Could you check a few things on this drawing? It's one solid part, dimensions in mm from its lowest x, y, z. Give positions to 0.01 mm unless a question says otherwise; leave off trailing zeros. Order: outer loops, then holes, each group sorted by start corner. A loop starts at its lowest first (then second) coordinate and runs counter-clockwise, first axis right, second up. Notation, with made-up numbers: (69.5, 22.5) -> (93.5, 22.5) arc R23 ccw to (93.5, 30.5) -> close; hole circle Ø8 at (-35.75, 69.25). An arc over 180 degrees is marked (long way). Answer as a JSON object with one key per item and string values.
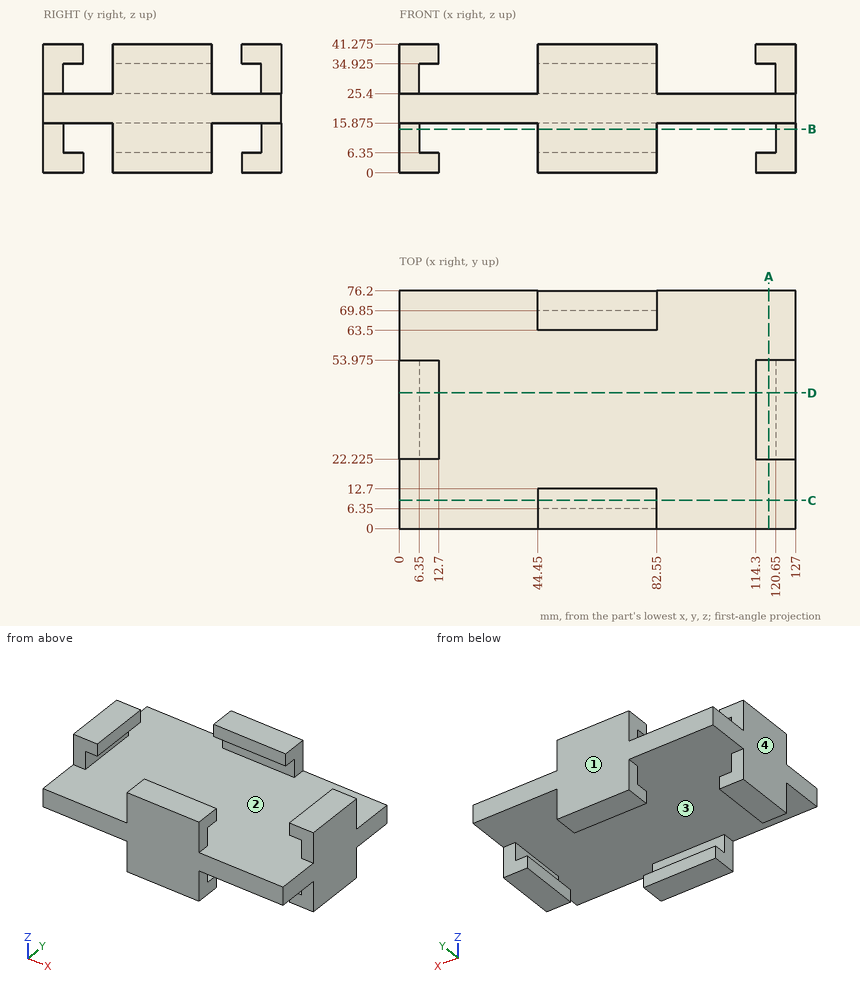
1. Will these pins go through, and if not, where does the flat tip stop? pin 1 Ø2 at (x, y) = (48, 34) entering from -Z (3 decimals); pin 2 Ø6 at (y, z) = (12, 8) entering from -X; pin 3 Ø14 at (x, z) = (9.5, 37) entering from +Y (3 decimals).
Worked answers:
{"pin 1": "z = 15.875", "pin 2": "x = 44.45", "pin 3": "y = 53.975"}
2. If we section it at A-A on x = 118.5: Please give me the cut outline in (y, z) (3 decimals).
Worked answers:
{"outline": "(0, 15.875) -> (76.2, 15.875) -> (76.2, 25.4) -> (0, 25.4) -> close; (22.225, 0) -> (53.975, 0) -> (53.975, 6.35) -> (22.225, 6.35) -> close; (22.225, 34.925) -> (53.975, 34.925) -> (53.975, 41.275) -> (22.225, 41.275) -> close"}
3. If we mould it in two halves opening along X, with no side actions, what happens to the marked faces 1, 2, 3 and 4? For each: +X half, -X half, draft (parallel to the pull), parting line (faces both ways), or undercut.
Worked answers:
{"face 1": "draft", "face 2": "undercut", "face 3": "undercut", "face 4": "-X half"}
4. If we section it at C-C on y = 9: Please give me the cut outline in (x, z) (3 decimals).
Worked answers:
{"outline": "(0, 15.875) -> (127, 15.875) -> (127, 25.4) -> (0, 25.4) -> close; (44.45, 0) -> (82.55, 0) -> (82.55, 6.35) -> (44.45, 6.35) -> close; (44.45, 34.925) -> (82.55, 34.925) -> (82.55, 41.275) -> (44.45, 41.275) -> close"}
5. If we section it at B-B on z = 14: Please give me the cut outline in (x, y) (3 decimals).
Worked answers:
{"outline": "(0, 22.225) -> (6.35, 22.225) -> (6.35, 53.975) -> (0, 53.975) -> close; (44.45, 0) -> (82.55, 0) -> (82.55, 6.35) -> (44.45, 6.35) -> close; (44.45, 69.85) -> (82.55, 69.85) -> (82.55, 76.2) -> (44.45, 76.2) -> close; (120.65, 22.225) -> (127, 22.225) -> (127, 53.975) -> (120.65, 53.975) -> close"}
6. If we section it at D-D on y = 43.5: Please give me the cut outline in (x, z) (3 decimals).
Worked answers:
{"outline": "(0, 0) -> (12.7, 0) -> (12.7, 6.35) -> (6.35, 6.35) -> (6.35, 15.875) -> (120.65, 15.875) -> (120.65, 6.35) -> (114.3, 6.35) -> (114.3, 0) -> (127, 0) -> (127, 41.275) -> (114.3, 41.275) -> (114.3, 34.925) -> (120.65, 34.925) -> (120.65, 25.4) -> (6.35, 25.4) -> (6.35, 34.925) -> (12.7, 34.925) -> (12.7, 41.275) -> (0, 41.275) -> close"}
7. Please list where these lines run through material, in increasing order: L1, parallel to Z at x = 53.5, y = 9 (3 decimals); L2, parallel to Y at x = 79, z = 34; L3, parallel to X at y = 46, z = 15.5.
Worked answers:
{"L1": "0 to 6.35, 15.875 to 25.4, 34.925 to 41.275", "L2": "0 to 6.35, 69.85 to 76.2", "L3": "0 to 6.35, 120.65 to 127"}
